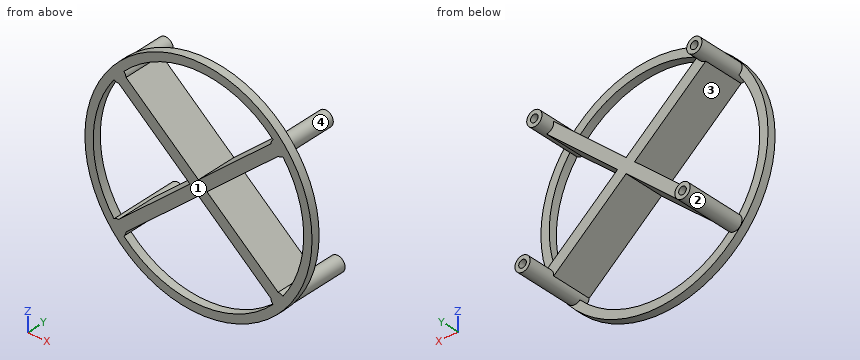
Autodesk Fusion 360 part; units mm, degrees
sketch "Sketch1" plane through (0, 0, 0) normal (0, 1, 0) x (1, 0, 0)
  circle A0 centre (0, 0) radius 44
  line L0 (28.875, 24.875) -> (-28.875, 24.875) construction
  line L1 (-28.875, 24.875) -> (-28.875, -24.875) construction
  line L2 (-28.875, -24.875) -> (28.875, -24.875) construction
  line L3 (28.875, -24.875) -> (28.875, 24.875) construction
  line L4 (28.875, 24.875) -> (-28.875, -24.875) construction
  line L5 (-28.875, 24.875) -> (28.875, -24.875) construction
  circle A1 centre (-28.875, 24.875) radius 1.375
  circle A2 centre (-28.875, 24.875) radius 2.75
  circle A3 centre (-28.875, -24.875) radius 1.375
  circle A4 centre (-28.875, -24.875) radius 2.75
  circle A5 centre (28.875, 24.875) radius 1.375
  circle A6 centre (28.875, 24.875) radius 2.75
  circle A7 centre (28.875, -24.875) radius 1.375
  circle A8 centre (28.875, -24.875) radius 2.75
  line L6 (-30.4443, 23.5871) -> (27.8036, -26.5919)
  line L7 (-27.8037, 26.5919) -> (30.4442, -23.5871)
  line L8 (27.8041, 26.5923) -> (-30.4447, -23.5875)
  line L9 (30.4447, 23.5875) -> (-27.8041, -26.5923)
  circle A9 centre (0, 0) radius 40.9963
  circle A10 centre (0, 0) radius 37.9963
  dimension "d1" = 88
  dimension "d2" = 57.75
  dimension "d3" = 49.75
  dimension "d4" = 2.75
  dimension "d5" = 5.5
  dimension "d6" = 2.75
  dimension "d7" = 5.5
  dimension "d8" = 2.75
  dimension "d9" = 5.5
  dimension "d10" = 2.75
  dimension "d11" = 5.5
  dimension "d26" = 2
  dimension "d27" = -2
  dimension "d28" = 2
  dimension "d29" = -2
  dimension "d30" = -3
extrude "Extrude1" add sketch "Sketch1" along normal blind 3 contours A0 | A1 A10 | A1 A2 L6 L7 A10 | A1 A10 | A1 A2 A10 | A2 L7 A10 | A2 L6 A10 | A2 L6 L7 L8 | A2 A6 L7 L8 A10 | A2 A4 L6 L8 A10 | A6 L7 L8 L9 | L6 L7 L8 L9 | A6 L8 A10 | A5 A6 A10 | A4 L6 L8 L9 | A3 A4 A10 | A4 L8 A10 | A6 A8 L7 L9 A10 | A8 L6 L7 L9 | A5 A6 L8 L9 A10 | A4 A8 L6 L9 A10 | A3 A4 L8 L9 A10 | A4 L9 A10 | A7 A8 L6 L7 A10 | A8 L7 A10 | A6 L9 A10 | A5 A10 | A5 A10 | A8 L6 A10 | A7 A8 A10 | A3 A10 | A3 A10 | A7 A10 | A7 A10 | A9 makes body 1
extrude "Extrude2" add sketch "Sketch1" along normal blind 20 contours A3 A4 A10 | A4 L8 A10 | A3 A4 L8 L9 A10 | A4 L9 A10 | A7 A8 L6 L7 A10 | A8 L7 A10 | A8 L6 A10 | A7 A8 A10 bodies 1
extrude "Extrude3" add sketch "Sketch1" along normal blind 25 contours A1 A2 L6 L7 A10 | A1 A2 A10 | A2 L7 A10 | A2 L6 A10 | A6 L8 A10 | A5 A6 A10 | A5 A6 L8 L9 A10 | A6 L9 A10 bodies 1
extrude "Extrude4" add sketch "Sketch1" along normal blind 15 contours A1 A10 | A1 A10 | A5 A10 | A5 A10 | A3 A10 | A3 A10 | A7 A10 | A7 A10 bodies 1
extrude "Extrude5" add sketch "Sketch1" along normal blind 15 contours A2 L6 L7 L8 | A6 L7 L8 L9 | L6 L7 L8 L9 | A4 L6 L8 L9 | A8 L6 L7 L9 bodies 1
extrude "Extrude7" add sketch "Sketch1" along normal blind 3 separate body contours A9 makes body 2
extrude "Extrude8" add sketch "Sketch1" along normal blind 15 separate body contours A1 A10 | A1 A10 | A2 L6 L7 L8 | A6 L7 L8 L9 | L6 L7 L8 L9 | A4 L6 L8 L9 | A8 L6 L7 L9 | A5 A10 | A5 A10 | A3 A10 | A3 A10 | A7 A10 | A7 A10 makes body 3 at (-27.5068, 10, -25.0119) makes body 4 at (30.2432, 5, -24.7381) makes body 5 at (-29.6776, 10, 25.9914) makes body 6 at (9.9096, 0, 8.6263) makes body 7 at (30.2432, 5, 25.0119)
extrude "Extrude9" add sketch "Sketch1" along normal blind 20 contours A3 A4 A10 | A4 L8 A10 | A3 A4 L8 L9 A10 | A4 L9 A10 | A7 A8 L6 L7 A10 | A8 L7 A10 | A8 L6 A10 | A7 A8 A10 bodies 2 5 6 7
extrude "Extrude10" add sketch "Sketch1" along normal blind 25 contours A1 A2 L6 L7 A10 | A1 A2 A10 | A2 L7 A10 | A2 L6 A10 | A6 L8 A10 | A5 A6 A10 | A5 A6 L8 L9 A10 | A6 L9 A10 bodies 2 3 4
hidden bodies 1
equation "d2 = 55 mm + 2.75 mm"
equation "d3 = 48 mm + 1.75 mm"
Can you work these out from the model? Positions are in its coordinate system, mm. Face numbers are marked on the shaded views. A direction names the side the tool comes from. Round coordinates to 2 decimals unless told otherwise and drop trailing zeros. Order: outer loops, then holes, each group sorted by start corner. A loop starts at its lowest first (then second) coordinate and runs counter-clockwise, first axis right, second up. Notation, with made-up numbers: M 56,-18.75 L 76,-18.75 A35 ccw 76,15.25 Z; hole C 83.25,88 d10. An arc over 180 degrees is marked long. Use a Markdown table: item, result.
1) Imagine slicing it at C-C (x = 8). List the corners of the cut face in (y, z) for me, then the cut area to 3 significant figures.
Geometry says:
| item | result |
|---|---|
| outline | M 0,-40.21 L 3,-40.21 L 3,-37.14 L 0,-37.14 Z; M 0,-9.53 L 15,-9.53 L 15,-4.25 L 0,-4.25 Z; M 0,4.25 L 15,4.25 L 15,9.53 L 0,9.53 Z; M 0,37.14 L 3,37.14 L 3,40.21 L 0,40.21 Z |
| area | 177 mm² |
2) I'm going to push flat-ended pins straight in: P1, Ø10, axis at x = -3.5, y = 17, coming from the -Z side; P2, Ø6, axis at y = 18, z = 29, coming from the -X side; P3, Ø4.5, axis at x = 27.5, z = 26, coming from the +Y side; P4, Ø2, axis at x = -29.5, z = -24.5, coming from the +Y side. Where does each tip first touch, or does it pass through?
Geometry says:
| item | result |
|---|---|
| P1 | stops at z = -9.6 |
| P2 | stops at x = -31.38 |
| P3 | stops at y = 20 |
| P4 | stops at y = 25 |
3) On a 3-axis mill with a long thin cutter (end or side, diameter ignored), from which of +Z, -Z, +X, -X, +Y, -Y can I reach the whole of each face in a straight line? I mean the marked faces 3 and 4. Say none if no direction works.
Geometry says:
| item | result |
|---|---|
| face 3 | +Y, -Y |
| face 4 | +Y |
4) Imagine slicing it at B-B (y = 4.25). List the corners of the cut face in (x, z) for me (3 decimals), then the cut area to 3 significant figures.
Geometry says:
| item | result |
|---|---|
| outline | M -28.75,-22.128 A2.75 ccw long -26.14,-25.158 L 0,-2.64 L 26.14,-25.158 A2.75 ccw long 28.75,-22.128 L 3.064,0 L 28.75,22.128 A2.75 ccw long 26.14,25.158 L 0,2.64 L -26.14,25.158 A2.75 ccw long -28.75,22.128 L -3.064,0 Z |
| area | 649 mm² |
5) Imagine slicing it at D-D (y = 23.5). List the corners of the cut face in (x, z) for me (3 decimals).
Geometry says:
| item | result |
|---|---|
| outline | C -28.875,-24.875 d5.5; C 28.875,-24.875 d5.5; hole C -28.875,-24.875 d2.75; hole C 28.875,-24.875 d2.75 |
6) If we mould it in two halves opening along Z, with no side actions, what happens to the marked faces 1 and 2? For each: +Z half, -Z half, draft (parallel to the pull), parting line (faces both ways), or undercut.
Geometry says:
| item | result |
|---|---|
| face 1 | draft |
| face 2 | undercut |
7) If I drill on line 1 along Y through (x, z) = (-16, -34.5); line 2 along Y through (x, z) = (1, 1.5); line 3 along Z through (x, y) = (25.5, 2.75), over which ranges is the centre line in solid material (lowest first)?
Geometry says:
| item | result |
|---|---|
| line 1 | y = 0 to 3 |
| line 2 | y = 0 to 15 |
| line 3 | z = -32.1 to -28.17, -24.61 to -19.33, 19.33 to 24.61, 28.17 to 32.1 |
8) Imagine slicing it at A-A (z = 19.5). List the corners of the cut face in (x, y) for me, then the cut area to 3 significant figures.
Geometry says:
| item | result |
|---|---|
| outline | M -36.06,0 L -32.61,0 L -32.61,3 L -36.06,3 Z; M -25.7,0 L -19.57,0 L -19.57,15 L -25.7,15 Z; M 19.57,0 L 25.7,0 L 25.7,15 L 19.57,15 Z; M 32.61,0 L 36.06,0 L 36.06,3 L 32.61,3 Z |
| area | 205 mm² |
